Part model, mm, in its own coordinate system. Face numbers are marked on the shaded views. A direction names the side the tool comes from. Give positions to 0.01 mm unless a question says otherwise; leave off trailing zeros.
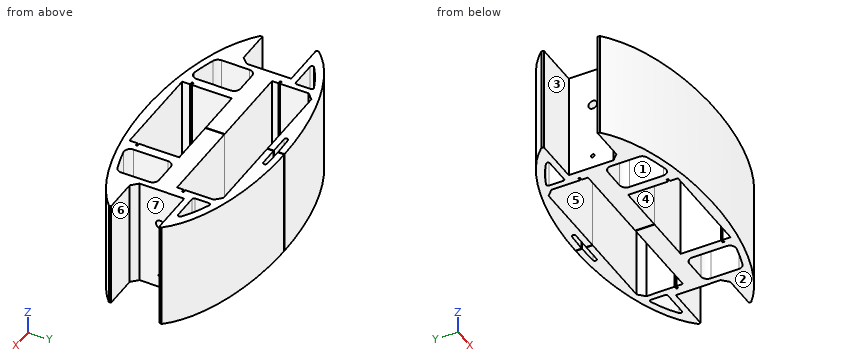
from build123d import *

# Parameters (mm, degrees)
SKETCH1_RX              = 244
SKETCH1_RY              = 110
BOSS_EXTRUDE1_DEPTH     = 170
SKETCH9_W               = 89
SKETCH9_H               = 81
CUT_EXTRUDE4_DEPTH      = 318.074123826
CUT_EXTRUDE5_DEPTH      = 307.853795271
CUT_EXTRUDE6_DEPTH      = 307.853795271
CUT_EXTRUDE6_DEPTH_BACK = 307.853795271
SKETCH11_R              = 6.83635542
SKETCH11_R_2            = 2.75
CHAMFER1_START          = -171
CHAMFER1_DEPTH          = 172
CUT_EXTRUDE7_DEPTH      = 305.55287031
CHAMFER2_SIZE           = 10
CUT_EXTRUDE8_DEPTH      = 305.55287031
CUT_EXTRUDE8_DEPTH_BACK = 305.55287031
SKETCH14_W              = 1
SKETCH14_H              = 125
CUT_EXTRUDE9_DEPTH      = 305.55287044
CUT_EXTRUDE9_DEPTH_BACK = 305.55287044
FILLET1_R               = 10
FILLET2_R               = 3
CHAMFER4_SIZE           = 10


with BuildPart() as part:
    # Sketch1 → Boss-Extrude1 (new body)
    with BuildSketch(Plane.XY):
        with Locations((0, 0)):
            Ellipse(SKETCH1_RX, SKETCH1_RY)
    extrude(amount=-BOSS_EXTRUDE1_DEPTH)

    # Sketch9 → Cut-Extrude4 (cut, through all)
    with BuildSketch(Plane.XY):
        with Locations((199.5, -4.5)):
            Rectangle(SKETCH9_W, SKETCH9_H)
        with Locations((-199.5, -4.5)):
            Rectangle(SKETCH9_W, SKETCH9_H)
    extrude(amount=-CUT_EXTRUDE4_DEPTH, mode=Mode.SUBTRACT)

    # Sketch10 → Cut-Extrude5 (cut, through all)
    with BuildSketch(Plane.XY):
        Polygon((-137.5, 83.1), (137.5, 83.1), (137.5, 28.1), (142.5, 28.1), (142.5, 25.1), (137.5, 25.1), (137.5, 15.1), (-137.5, 15.1), (-137.5, 25.1), (-142.5, 25.1), (-142.5, 28.1), (-137.5, 28.1), align=None)
    extrude(amount=-CUT_EXTRUDE5_DEPTH, mode=Mode.SUBTRACT)

    # Sketch11 → Cut-Extrude6 (cut, two sides: drawn at the far end of the back side and taken through both)
    with BuildSketch(Plane(origin=(0, 0, 0), x_dir=(0, 0, -1), z_dir=(1, 0, 0)).offset(-CUT_EXTRUDE6_DEPTH_BACK)):
        with Locations(Location((60, -2, 0), (0, 0, 270))):
            Circle(SKETCH11_R)
        with Locations(Location((150, -2, 0), (0, 0, 270))):
            Circle(SKETCH11_R_2)
    extrude(amount=CUT_EXTRUDE6_DEPTH + CUT_EXTRUDE6_DEPTH_BACK, mode=Mode.SUBTRACT)

    # Chamfer1: read off the stored shape, not the designer's step
    # Chamfer1 outline → Chamfer1 (cut)
    with BuildSketch(Plane.XY.offset(CHAMFER1_START)):
        with BuildLine():
            add(Edge.make_bspline(
                [(230.562901548, 36), (229.103745792, 37.899303194), (227.491649987, 39.773306403)],
                knots=[0.33341591, 0.33341591, 0.33341591, 0.380657268, 0.380657268, 0.380657268], degree=2, weights=[1, 0.987158133, 0.974806549]))
            Line((227.491649987, 39.773306403), (226.997134148, 36))
            Line((226.997134148, 36), (230.562901548, 36))
        make_face()
        with BuildLine():
            Line((-226.997134148, 36), (-227.491649987, 39.773306403))
            add(Edge.make_bspline(
                [(-227.491649987, 39.773306403), (-229.103745792, 37.899303194), (-230.562901548, 36)],
                knots=[2.760935386, 2.760935386, 2.760935386, 2.808176743, 2.808176743, 2.808176743], degree=2, weights=[0.974806549, 0.987158133, 1]))
            Line((-230.562901548, 36), (-226.997134148, 36))
        make_face()
        with BuildLine():
            add(Edge.make_bspline(
                [(-222.648446162, -45), (-220.94937929, -46.708532895), (-219.122315767, -48.390007394)],
                knots=[3.563050222, 3.563050222, 3.563050222, 3.605462156, 3.605462156, 3.605462156], degree=2, weights=[1, 0.989097384, 0.978597088]))
            Line((-219.122315767, -48.390007394), (-219.112898615, -45))
            Line((-219.112898615, -45), (-222.648446162, -45))
        make_face()
        with BuildLine():
            Line((219.112898615, -45), (219.122315767, -48.390007394))
            add(Edge.make_bspline(
                [(219.122315767, -48.390007394), (220.94937929, -46.708532895), (222.648446162, -45)],
                knots=[5.819315805, 5.819315805, 5.819315805, 5.861727739, 5.861727739, 5.861727739], degree=2, weights=[0.978597088, 0.989097384, 1]))
            Line((222.648446162, -45), (219.112898615, -45))
        make_face()
    extrude(amount=CHAMFER1_DEPTH, mode=Mode.SUBTRACT)

    # Sketch13 → Cut-Extrude7 (cut, through all)
    with BuildSketch(Plane.XY):
        Polygon((-76.2, -81.5), (-76.2, -93.9), (76.2, -93.9), (76.2, -81.5), (81.2, -81.5), (81.2, -78.5), (76.2, -78.5), (76.2, -15), (-76.2, -15), (-76.2, -78.5), (-81.2, -78.5), (-81.2, -81.5), align=None)
    extrude(amount=-CUT_EXTRUDE7_DEPTH, mode=Mode.SUBTRACT)

    # Chamfer2
    chamfer2_edges = [part.edges().sort_by_distance(p)[0] for p in [
        (155, -45, -85),
        (-155, -45, -85),
    ]]
    chamfer(chamfer2_edges, length=CHAMFER2_SIZE)

    # Sketch14 → Cut-Extrude8 (cut, two sides: drawn at the far end of the back side and taken through both)
    with BuildSketch(Plane.XY.offset(-CUT_EXTRUDE8_DEPTH_BACK)):
        with Locations((0, 47.5)):
            Rectangle(SKETCH14_W, SKETCH14_H)
    extrude(amount=CUT_EXTRUDE8_DEPTH + CUT_EXTRUDE8_DEPTH_BACK, mode=Mode.SUBTRACT)

    # Sketch15 → Cut-Extrude9 (cut, two sides: drawn at the far end of the back side and taken through both)
    with BuildSketch(Plane.XY.offset(-CUT_EXTRUDE9_DEPTH_BACK)):
        with BuildLine():
            Line((147.5, 75.514694834), (147.5, 46))
            Line((147.5, 46), (199.781755924, 46))
            add(Edge.make_bspline(
                [(199.781755924, 46), (179.990233789, 62.979001801), (147.5, 75.514694834)],
                knots=[3.619587852, 3.619587852, 3.619587852, 3.997470903, 3.997470903, 3.997470903], degree=2, weights=[1, 0.982203587, 1]))
        make_face()
        with BuildLine():
            Line((91.2, -91.41689608), (91.2, -15))
            Line((91.2, -15), (145, -15))
            Line((145, -15), (145, -76.465113485))
            add(Edge.make_bspline(
                [(91.2, -91.41689608), (120.495747781, -85.643811522), (145, -76.465113485)],
                knots=[1.988139758, 1.988139758, 1.988139758, 2.27109284, 2.27109284, 2.27109284], degree=2, weights=[1, 0.990008876, 1]))
        make_face()
        with BuildLine():
            Line((-82.129314955, 93.1), (82.129314955, 93.1))
            add(Edge.make_bspline(
                [(82.129314955, 93.1), (0, 107.411385607), (-82.129314955, 93.1)],
                knots=[4.338735578, 4.338735578, 4.338735578, 5.086042382, 5.086042382, 5.086042382], degree=2, weights=[1, 0.931, 1]))
        make_face()
        with BuildLine():
            Line((-91.2, -91.41689608), (-91.2, -15))
            Line((-91.2, -15), (-145, -15))
            Line((-145, -15), (-145, -76.465113485))
            add(Edge.make_bspline(
                [(-145, -76.465113485), (-120.495747781, -85.643811522), (-91.2, -91.41689608)],
                knots=[0.870499814, 0.870499814, 0.870499814, 1.153452896, 1.153452896, 1.153452896], degree=2, weights=[1, 0.990008876, 1]))
        make_face()
        with BuildLine():
            Line((-147.5, 75.514694834), (-147.5, 46))
            Line((-147.5, 46), (-199.781755924, 46))
            add(Edge.make_bspline(
                [(-147.5, 75.514694834), (-179.990233789, 62.979001801), (-199.781755924, 46)],
                knots=[5.427307058, 5.427307058, 5.427307058, 5.805190109, 5.805190109, 5.805190109], degree=2, weights=[1, 0.982203587, 1]))
        make_face()
    extrude(amount=CUT_EXTRUDE9_DEPTH + CUT_EXTRUDE9_DEPTH_BACK, mode=Mode.SUBTRACT)

    # Fillet1
    fillet1_edges = [part.edges().sort_by_distance(p)[0] for p in [
        (-145, -15, -85),
        (-145, -76.465113485, -85),
        (-91.2, -91.41689608, -85),
        (145, -76.465113485, -85),
        (91.2, -91.41689608, -85),
        (91.2, -15, -85),
        (-91.2, -15, -85),
        (145, -15, -85),
    ]]
    fillet(fillet1_edges, radius=FILLET1_R)

    # Fillet2
    fillet2_edges = [part.edges().sort_by_distance(p)[0] for p in [
        (-82.129314955, 93.1, -85),
        (82.129314955, 93.1, -85),
        (199.781755924, 46, -85),
        (147.5, 75.514694834, -85),
        (147.5, 46, -85),
        (-147.5, 75.514694834, -85),
        (-147.5, 46, -85),
        (-199.781755924, 46, -85),
    ]]
    fillet(fillet2_edges, radius=FILLET2_R)

    # Chamfer4
    chamfer4_edges = [part.edges().sort_by_distance(p)[0] for p in [
        (-137.5, 83.1, -85),
        (137.5, 83.1, -85),
    ]]
    chamfer(chamfer4_edges, length=CHAMFER4_SIZE)


solid = part.part
1) Mould opens along X. For the marked faces 4, 5, 6 and 7 say: +X half, -X half, draft (parallel to the pull), parting line (faces both ways), or undercut.
Check result:
face 4: undercut
face 5: undercut
face 6: draft
face 7: +X half
2) Saw through at A-A (z = -60). State how many separate pieces and enclosed holes the cut face has, and give its area (3 significant figures).
Check result:
separate pieces: 3
enclosed holes: 4
area: 26,500 mm2
3) Drill centre lines: L1, parallel to Z at x = 44, y = -2; L2, parallel to X at y = -48, z = -115; L3, parallel to Y at x = 72, z = -150. Where is each one in solid material? Low to high.
Check result:
L1: z = -170 to -152.75, -147.25 to -66.84, -53.16 to 0
L2: x = -219.12 to -145, -91.2 to -76.2, 76.2 to 91.2, 145 to 219.12
L3: y = -105.1 to -93.9, -15 to -4.75, 0.75 to 15.1, 83.1 to 105.1
4) Flat gauge pins, fed straight in: P1, Ø3, axis at y = -35.5, z = -62, coming from the -X side; P2, Ø3.5, axis at y = 27, z = -72.5, coming from the +X side; P3, Ø1.5, axis at y = -80, z = -121, coming from the -X side. Where does each tip first touch, or does it go through?
Check result:
P1: stops at x = -157
P2: stops at x = 155
P3: stops at x = -169.21
5) 3-axis set-ups, long thin cutter, end or side, ignore diameter. For the marked faces 1, 2 and 3: which of +Z, -Z, +X, -X, +Y, -Y reach the whole face in a straight line?
Check result:
face 1: +Z, -Z
face 2: -Z, +X, -X, +Y, -Y
face 3: +Z, -Z, -X
